The model under review builds one solid part; all positions refer to its coordinate system, in mm. A direction names the side the tool comes from. Coordinates: 2 decimals unless noted, no trailing zeros. Write each loop counter-clockwise with the first axis right and the second up, starting at its lowest first coordinate (ties: lowest second). Pieces come first, ordered by that corner, then holes. Notation, with made-up numbers: (-27.5, 25) - (-0.5, 25) arc R18 ccw to (-0.5, 49) - close; hole circle Ø9 at (17, -5.75). An arc over 180 degrees is marked (long way). Return JSON: item names as keys, results as strings. Group by question number.
(1) Draft analysis for pull direction X (two halves, no side actions). For faces 1 (the face through (32.589, -45, 13)), 2 (the face through (-15.225, -93.563, 12.522)), 3 (the face through (-113.445, -70, 13)), 4 (the face through (-84, -20.428, 13)), state which applies: released by +X, released by -X, zero draft, split by the parting line, or undercut.
(2) For pin 1 Ø12.5 at (x, z) = (-85, 14) entering from +Y; pin 2 Ø5 at (x, z) = (-55, 13.5) entering from -Y; pin 3 Ø10 at (x, y) = (-12.5, -41) entering from +Z; pin 4 Ø1.5 at (y, z) = (-91, 4) entering from +X, all flat-tipped, find the tip position at first contact; note any pin that passes through.
(3) To check wall thickness, follow L1, parallel to X at y = -65.5, z = 17; L2, parallel to X at y = -40, z = 16.5; L3, parallel to X at y = -5.5, z = 9. State the ranges of each line that lie inside material, in increasing order. Write a range as from..to.
(4) We need section A-A on x = -0.5. State the section outline as (y, z) points.
(5) We need section B-B on y = -49. State the section outline as (x, z) points.
(6) We need section D-D on z = 6. Give the number of separate pieces and of enclosed holes in the cut face, then the cut area to 3 significant figures.
(7) Tool access review of faces 5 (the face through (-98.3, -40.6, 12.5)), 6 (the face through (-35.7, -81.1, 12.5)): name each direction out of +Z, -Z, +X, -X, +Y, -Y from which nothing blocks a thin tool from reaching the whole face with its end or side.
(8) We need section C-C on y = -86.5. State the section outline as (x, z) points.
```python
from build123d import *

# Parameters (mm, degrees)
F2_DEPTH = 25.4


# Not quite as in the source:
# - the program builds the solid bodies; features that only make, move or delete a surface that nothing else refers to are left out


with BuildPart() as f2:
    # F0 (on Top) → F2 (new body)
    with BuildSketch(Plane.XY):
        with BuildLine():
            ThreePointArc((-105.2959337831, -13.8524966314), (-110.9424227524, -15.1925239823), (-113.4453713894, -20.4283390194))
            Line((-113.4453713894, -20.4283390194), (-113.4453713894, -120.5272600055))
            ThreePointArc((-113.4453713894, -120.5272600055), (-106.8133786321, -124.9365702093), (-100.1813858747, -120.5272600055))
            Line((-100.1813858747, -120.5272600055), (-100.1813858747, -99.1557762027))
            ThreePointArc((-100.1813858747, -99.1557762027), (-98.8733273351, -96.1822516833), (-95.7974940538, -95.1372087002))
            Line((-95.7974940538, -95.1372087002), (-66.7541921139, -95.1372087002))
            ThreePointArc((-66.7541921139, -95.1372087002), (-53.508361005, -88.6629146032), (-42.6427721977, -78.6975994706))
            Line((-42.6427721977, -78.6975994706), (-40.7650305092, -76.3982318447))
            Line((-40.7650305092, -76.3982318447), (-37.9493655476, -78.6975994706))
            Line((-37.9493655476, -78.6975994706), (-33.326998353, -83.6294814944))
            Line((-33.326998353, -83.6294814944), (-27.1164793521, -88.1960391998))
            Line((-27.1164793521, -88.1960391998), (-20.3579775989, -92.0319482684))
            Line((-20.3579775989, -92.0319482684), (-9.9462270737, -95.1372087002))
            Line((-9.9462270737, -95.1372087002), (-1.5437625116, -95.1372087002))
            Line((-1.5437625116, -95.1372087002), (11.6079188883, -95.1372087002))
            Line((11.6079188883, -95.1372087002), (18.3664243668, -95.1372087002))
            ThreePointArc((18.3664243668, -95.1372087002), (21.0049540589, -98.8169422623), (24.7596036643, -101.3477295637))
            ThreePointArc((24.7596036643, -101.3477295637), (30.3769038734, -100.3890234282), (32.5886048377, -95.1372087002))
            Line((32.5886048377, -95.1372087002), (32.5886048377, -83.264157176))
            Line((32.5886048377, -83.264157176), (32.5886048377, -36.867942661))
            Line((32.5886048377, -36.867942661), (32.5886048377, 6.9710011594))
            ThreePointArc((32.5886048377, 6.9710011594), (26.2081623077, 9.0786866715), (19.8277197778, 6.9710011594))
            Line((19.8277197778, 6.9710011594), (19.8277197778, -17.5057426095))
            ThreePointArc((19.8277197778, -17.5057426095), (18.7722789641, -19.7743587388), (16.3571424782, -20.4283390194))
            Line((16.3571424782, -20.4283390194), (-11.9555136189, -20.4283390194))
            ThreePointArc((-11.9555136189, -20.4283390194), (-27.5905728803, -27.3736232216), (-40.0855019689, -39.0598885715))
            ThreePointArc((-40.0855019689, -39.0598885715), (-53.2554420129, -27.1621160119), (-69.6767866611, -20.4283390194))
            Line((-69.6767866611, -20.4283390194), (-99.268078804, -20.4283390194))
            ThreePointArc((-99.268078804, -20.4283390194), (-101.8637236034, -16.7569920607), (-105.2959337831, -13.8524966314))
        make_face()
        with BuildLine():
            ThreePointArc((-94.1535308957, -35.954631865), (-64.4908309504, -37.7586891963), (-47.9399785399, -62.4406598508))
            ThreePointArc((-47.9399785399, -62.4406598508), (-57.037773934, -73.3713012414), (-69.5008059195, -80.2212381733))
            Line((-69.5008059195, -80.2212381733), (-88.1256759167, -81.2548696995))
            ThreePointArc((-88.1256759167, -81.2548696995), (-94.899092444, -79.4350063569), (-99.268078804, -73.9483833313))
            Line((-99.268078804, -73.9483833313), (-99.268078804, -46.5490445495))
            ThreePointArc((-99.268078804, -46.5490445495), (-98.2570203257, -40.5053887944), (-94.1535308957, -35.954631865))
        make_face(mode=Mode.SUBTRACT)
        with BuildLine():
            ThreePointArc((-30.4044019431, -51.2982606888), (-20.909712223, -39.8003863828), (-6.8409675732, -34.8586589098))
            Line((-6.8409675732, -34.8586589098), (8.6853252724, -34.8586589098))
            ThreePointArc((8.6853252724, -34.8586589098), (16.4998756565, -38.1334471627), (19.6450613439, -46.0010543466))
            Line((19.6450613439, -46.0010543466), (19.6450613439, -69.3818256259))
            ThreePointArc((19.6450613439, -69.3818256259), (16.328027351, -77.3898536128), (8.3199990913, -80.7068869472))
            Line((8.3199990913, -80.7068869472), (-9.5809019141, -80.7068854751))
            ThreePointArc((-9.5809019141, -80.7068854751), (-23.6431681808, -72.6575432123), (-32.5963497162, -59.1527372599))
            ThreePointArc((-32.5963497162, -59.1527372599), (-31.6935007339, -55.171603632), (-30.4044019431, -51.2982606888))
        make_face(mode=Mode.SUBTRACT)
    extrude(amount=F2_DEPTH)


solid = f2.part
```
Ans:
{
 "1": {"face 1": "released by +X", "face 2": "undercut", "face 3": "released by -X", "face 4": "undercut"},
 "2": {"pin 1": "y = -20.43", "pin 2": "y = -91.13", "pin 3": "z = 25.4", "pin 4": "x = 32.59"},
 "3": {"L1": "-113.45..-99.27, -49.83..-29.5, 19.65..32.59", "L2": "-113.45..-98, -61.08..-21.19, 17.97..32.59", "L3": "19.83..32.59"},
 "4": {"outline": "(-95.14, 0) - (-80.71, 0) - (-80.71, 25.4) - (-95.14, 25.4) - close; (-34.86, 0) - (-20.43, 0) - (-20.43, 25.4) - (-34.86, 25.4) - close"},
 "5": {"outline": "(-113.45, 0) - (-99.27, 0) - (-99.27, 25.4) - (-113.45, 25.4) - close; (-52.78, 0) - (-29.25, 0) - (-29.25, 25.4) - (-52.78, 25.4) - close; (19.65, 0) - (32.59, 0) - (32.59, 25.4) - (19.65, 25.4) - close"},
 "6": {"separate pieces": "1", "enclosed holes": "2", "area": "6,980 mm²"},
 "7": {"face 5": "+Z, -Z", "face 6": "+Z, -Z, -Y"},
 "8": {"outline": "(-113.45, 0) - (-50.57, 0) - (-50.57, 25.4) - (-113.45, 25.4) - close; (-29.42, 0) - (32.59, 0) - (32.59, 25.4) - (-29.42, 25.4) - close"}
}
